Source: CAD feature listing. Evaluate the final solid. Frame: model axes, mm. Face numbers are marked on the shaded views. A direction names the side the tool comes from. Coordinates: 2 decimals unless noted, no trailing zeros. Loops run counter-clockwise (first coordinate to the right, second up) from the corner with the lowest first, then second, coordinate; pieces in that order, holes last.
Item 1: Line query: probe 1 along Z at (x, y) = (79.5, -12) (3 decimals); probe 2 along Z at (x, y) = (49.5, -14.25) (3 decimals). Output: solid intervals per line, ascending.
Item 2: Pin query (flat end, axial travel): pin 1 Ø1 at (x, z) = (8.5, 41) entering from +Y; pin 2 Ø2 at (x, y) = (8.5, -15) entering from -Z. Return the tip coordinate at first contact, or that it passes through.
Item 3: Section query B-B, the plane x = 29. Return the cut outline in (y, z) (3 decimals), then the cut area to 3 significant figures.
Item 4: Reachability of the marked faces 1, 2 and 3 from +Z, -Z, +X, -X, +Y, -Y: full face, straight path, thin tool, end or side. Return the list, or none.
Item 5: Section query A-A, the plane y = -5.5. Return the cut outline in (x, z) (3 decimals).
```python
from build123d import *

# Parameters (mm, degrees)
F0_W     = 138.4305804968
F0_H     = 49.4050085545
F1_DEPTH = 25.4
F2_R     = 17.004974152
F3_DEPTH = 25.4


# Not quite as in the source:
# - the program builds the solid bodies; features that only make, move or delete a surface that nothing else refers to are left out


with BuildPart() as f1:
    # F0 (on Front) → F1 (new body)
    with BuildSketch(Plane.XZ):
        with Locations((52.0747005939, 24.7025042772)):
            Rectangle(F0_W, F0_H)
    extrude(amount=F1_DEPTH)

    # F2 (on Front) → F3 (join)
    with BuildSketch(Plane.XZ):
        with Locations((56.1164021492, 13.9775313437)):
            Circle(F2_R)
    extrude(amount=F3_DEPTH)


solid = f1.part
```
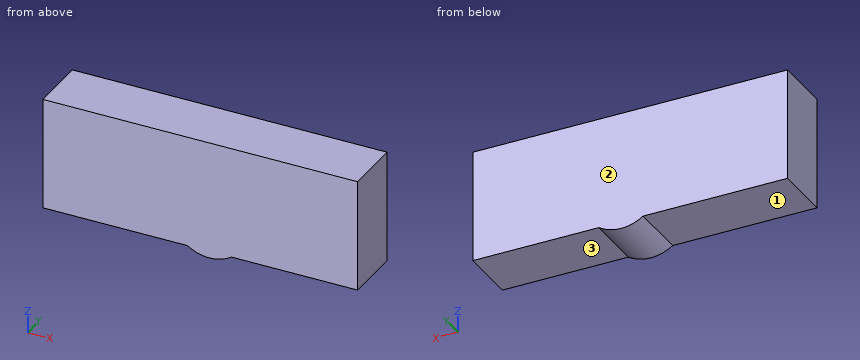
Verdict:
1. probe 1: z = 0 to 49.405
1. probe 2: z = -1.687 to 49.405
2. pin 1: stops at y = 0
2. pin 2: stops at z = 0
3. outline: (-25.4, 0) - (0, 0) - (0, 49.405) - (-25.4, 49.405) - close
3. area: 1,250 mm2
4. face 1: -Z, -X, +Y, -Y
4. face 2: +Z, -Z, +X, -X, +Y
4. face 3: -Z, +X, +Y, -Y
5. outline: (-17.141, 0) - (46.431, 0) arc R17.005 ccw to (65.801, 0) - (121.29, 0) - (121.29, 49.405) - (-17.141, 49.405) - close
